```python
from build123d import *

# Parameters (mm, degrees)
SKIZZE1_R                       = 16.75
SKIZZE1_R_2                     = 4.2
SKIZZE1_W                       = 9.6
SKIZZE1_H                       = 9.6
AUFSATZ_LINEAR_AUSTRAGEN1_DEPTH = 9.6
VERRUNDUNG1_R                   = 1


with BuildPart() as part:
    # Skizze1 → Aufsatz-Linear austragen1 (new body)
    with BuildSketch(Plane(origin=(0, 0, 0), x_dir=(1, 0, 0), z_dir=(0, 1, 0))):
        with Locations(Location((0, 0, 0), (0, 0, 270))):
            Circle(SKIZZE1_R)
        with Locations(Location((0, 0, 0), (0, 0, 270))):
            Circle(SKIZZE1_R_2, mode=Mode.SUBTRACT)
        with Locations((0, 10)):
            Rectangle(SKIZZE1_W, SKIZZE1_H, mode=Mode.SUBTRACT)
        with Locations((10, 0)):
            Rectangle(SKIZZE1_W, SKIZZE1_H, mode=Mode.SUBTRACT)
        with Locations((0, -10)):
            Rectangle(SKIZZE1_W, SKIZZE1_H, mode=Mode.SUBTRACT)
        with Locations((-10, 0)):
            Rectangle(SKIZZE1_W, SKIZZE1_H, mode=Mode.SUBTRACT)
    extrude(amount=AUFSATZ_LINEAR_AUSTRAGEN1_DEPTH)

    # Verrundung1
    verrundung1_edges = [part.edges().sort_by_distance(p)[0] for p in [
        (0, 0, -4.2),
        (0, 9.6, -4.2),
        (0, 0, -16.75),
        (0, 9.6, -16.75),
    ]]
    fillet(verrundung1_edges, radius=VERRUNDUNG1_R - 0.0001)  # a hair under: the kernel refuses the full size


solid = part.part
```
Here's how the part is built. I have some questions about the finished solid (model axes, mm). A direction names the side the tool comes from. Coordinates: 2 decimals unless noted, no trailing zeros. Loops run counter-clockwise (first coordinate to the right, second up) from the corner with the lowest first, then second, coordinate; pieces in that order, holes last. Notation, with made-up numbers: (3, 21) - (24, 21) arc R12 ccw to (24, 26) - close; hole circle Ø4 at (-39, 26). An arc over 180 degrees is marked (long way). Return JSON: item names as keys, results as strings. Group by question number.
Item 1: Will these pins go through, and if not, where does the flat tip stop? P1, Ø5, axis at y = 5.5, z = -10.5, coming from the +X side; P2, Ø1, axis at x = -4, y = 2.5, coming from the -Z side; P3, Ø5, axis at y = 3, z = 9.5, coming from the +X side.
Item 2: If we section it at A-A on x = 0: State how many separate pieces and enclosed holes the cut face has, and give its area (3 significant figures).
Item 3: On a 3-axis mill with a long thin cutter (end or side, diameter ignored), from which of +Z, -Z, +X, -X, +Y, -Y can I reach the whole of each face in a straight line? I mean faces 1 (the face through (-2, 0, -5)), 2 (the face through (4.8, 5, 10)). Say none if no direction works.
Item 4: I need wall thicknesses on line 1 (X direction, y = 5.5, z = 0); line 2 (X direction, y = 3, z = -10); line 3 (X direction, y = 9, z = -1.5). Which ranges of each line are inside material? Lowest first, please. Write a range as from..to.
Item 5: We'd pull the mould along Z, two halves only. Please class faces 3 (the face through (4.8, 5, -10)), 4 (the face through (-2, 9.6, -5)), 5 (the face through (-14.86, 4.75, 7.73)): +Z half, -Z half, draft (parallel to the pull), parting line (faces both ways), or undercut.
Item 6: If we section it at C-C on y = 7: Write out the boundary of the cut face in (x, z).
Calculated:
{
 "1": {"P1": "stops at x = 14.72", "P2": "stops at z = -16.38", "P3": "stops at x = 15.22"},
 "2": {"separate pieces": "4", "enclosed holes": "0", "area": "54.9 mm^2"},
 "3": {"face 1": "+Z, -Z, +X, -X, -Y", "face 2": "+Y, -Y"},
 "4": {"line 1": "x = -16.75..-14.8, -5.2..-4.2, 4.2..5.2, 14.8..16.75", "line 2": "x = -13.44..-4.8, 4.8..13.44", "line 3": "x = -16.6..-14.8, -5.2..-4.01, 4.01..5.2, 14.8..16.6"},
 "5": {"face 3": "undercut", "face 4": "draft", "face 5": "parting line"},
 "6": {"outline": "circle Ø33.5 at (0, 0); hole (-14.8, -4.8) - (-5.2, -4.8) - (-5.2, 4.8) - (-14.8, 4.8) - close; hole (-4.8, -14.8) - (4.8, -14.8) - (4.8, -5.2) - (-4.8, -5.2) - close; hole (-4.8, 5.2) - (4.8, 5.2) - (4.8, 14.8) - (-4.8, 14.8) - close; hole circle Ø8.4 at (0, 0); hole (5.2, -4.8) - (14.8, -4.8) - (14.8, 4.8) - (5.2, 4.8) - close"}
}
